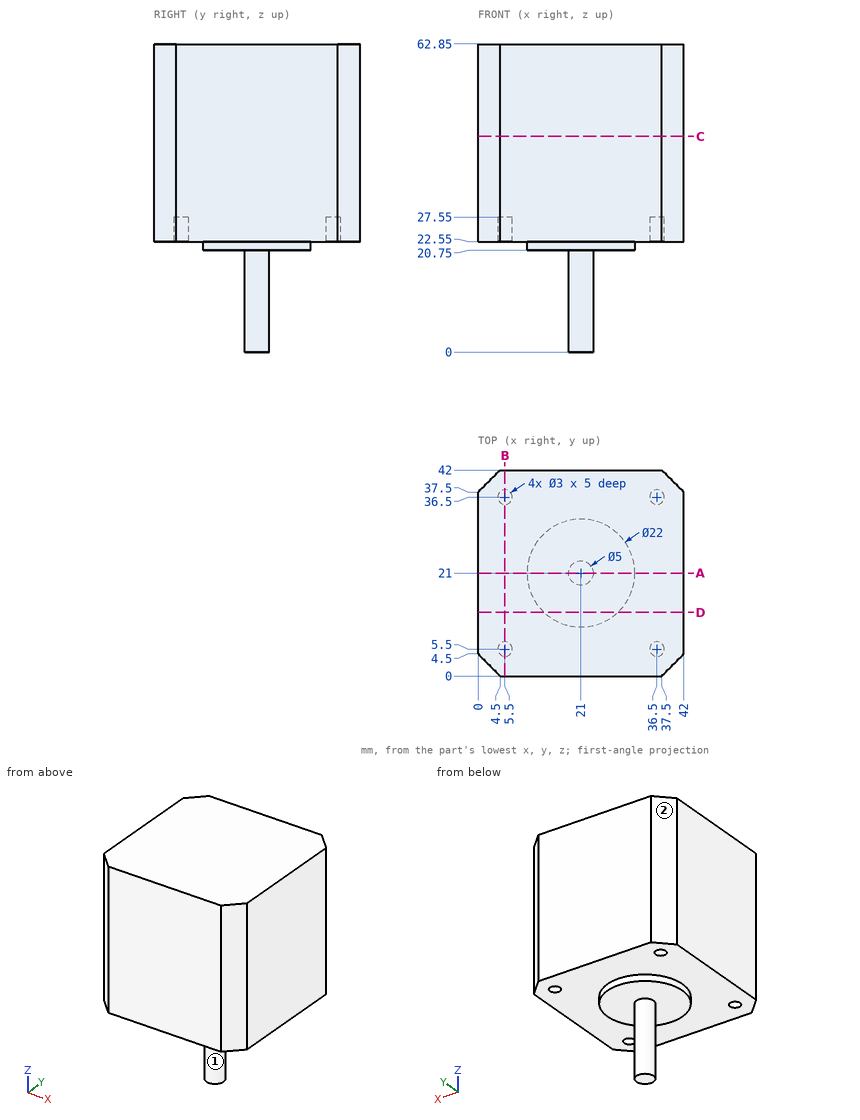
Here's the drawing with two shaded views (mm, measured from the low corner). I have some questions. A direction names the side the tool comes from. Give positions to 0.01 mm unless a question says otherwise; leave off trailing zeros. Write each loop counter-clockwise with the first axis right and the second up, starting at its lowest first coordinate (ties: lowest second). Pieces come first, ordered by that corner, then holes. Notation, with made-up numbers: (81, 37) -> (133, 37) arc R22 cw to (133, 74) -> close; hole circle Ø5 at (63, -39). An arc over 180 degrees is marked (long way). Answer as a JSON object with one key per item and string values. Group by question number.
Item 1: Please list where these lines run through material, in increasing order: line 1 (Y direction, x = 5.5, z = 23.75); line 2 (X direction, y = 5, z = 24). Write a range as [from, to].
Item 2: Suppose I cut it at C-C (z = 44). Please give me the cut outline in (x, y), plus the area to 3 significant figures.
Item 3: Suppose I cut it at A-A (y = 21). Please give me the cut outline in (x, z).
Item 4: Suppose I cut it at D-D (y = 13). Please give me the cut outline in (x, z), plus the area to 3 significant figures.
Item 5: For the marked faces 1 and 2, which set-ups out of +Z, -Z, +X, -X, +Y, -Y let a thin tool reach every point of the face, with its end or its side?
Item 6: Suppose I cut it at B-B (x = 5.5). Please give me the cut outline in (y, z).
Item 7: I'm going to push flat-ended pins straight in: P1, Ø5, axis at x = 36.5, y = 36.5, coming from the -Z side; P2, Ø1.5, axis at x = 5, y = 37, coming from the -Z side; P3, Ø1, axis at y = 28.5, z = 41.5, coming from the -X side; P4, Ø5, axis at x = 20.5, z = 20, coming from the +Y side. Where does each tip first touch, or does it pass through?
Findings:
{
 "1": {"line 1": "y = [0, 4], [7, 35], [38, 42]", "line 2": "x = [0, 4.09], [6.91, 35.09], [37.91, 42]"},
 "2": {"outline": "(0, 4.5) -> (4.5, 0) -> (37.5, 0) -> (42, 4.5) -> (42, 37.5) -> (37.5, 42) -> (4.5, 42) -> (0, 37.5) -> close", "area": "1,720 mm²"},
 "3": {"outline": "(0, 22.55) -> (10, 22.55) -> (10, 20.75) -> (18.5, 20.75) -> (18.5, 0) -> (23.5, 0) -> (23.5, 20.75) -> (32, 20.75) -> (32, 22.55) -> (42, 22.55) -> (42, 62.85) -> (0, 62.85) -> close"},
 "4": {"outline": "(0, 22.55) -> (13.45, 22.55) -> (13.45, 20.75) -> (28.55, 20.75) -> (28.55, 22.55) -> (42, 22.55) -> (42, 62.85) -> (0, 62.85) -> close", "area": "1,720 mm²"},
 "5": {"face 1": "-Z", "face 2": "+Z, -Z, -X, +Y"},
 "6": {"outline": "(0, 22.55) -> (4, 22.55) -> (4, 27.55) -> (7, 27.55) -> (7, 22.55) -> (35, 22.55) -> (35, 27.55) -> (38, 27.55) -> (38, 22.55) -> (42, 22.55) -> (42, 62.85) -> (0, 62.85) -> close"},
 "7": {"P1": "stops at z = 22.55", "P2": "stops at z = 27.55", "P3": "stops at x = 0", "P4": "stops at y = 32"}
}
